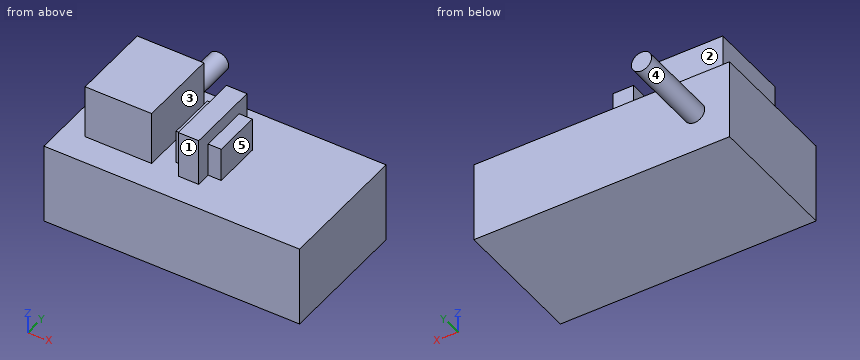
from build123d import *

# Parameters (mm, degrees)
F0_W     = 241.3
F0_H     = 76.2
F1_DEPTH = 127
F2_W     = 62.8207884729
F2_H     = 76.4612257481
F3_DEPTH = 50.8
F4_W     = 19.3203594536
F4_H     = 70.8669982851
F5_DEPTH = 44.45
F6_W     = 10.7880616561
F6_H     = 45.5669872463
F6_W_2   = 12.3340738937
F6_H_2   = 45.5182045698
F7_DEPTH = 31.75
F8_R     = 9.525
F9_DEPTH = 77.978


with BuildPart() as f1:
    # F0 (on Front) → F1 (new body)
    with BuildSketch(Plane.XZ):
        Rectangle(F0_W, F0_H)
    extrude(amount=-F1_DEPTH)

    # F2 (on face) → F3 (join)
    with BuildSketch(Plane.XY.offset(38.1)):
        with Locations((-68.2148206979, 66.0216137767)):
            Rectangle(F2_W, F2_H)
    extrude(amount=F3_DEPTH)

    # F4 (on face) → F5 (join)
    with BuildSketch(Plane.XY.offset(38.1)):
        with Locations((-0.7133577019, 61.1537639052)):
            Rectangle(F4_W, F4_H)
    extrude(amount=F5_DEPTH)

    # F6 (on face) → F7 (join)
    with BuildSketch(Plane.XY.offset(38.1)):
        with Locations((-15.7675682567, 62.2907597572)):
            Rectangle(F6_W, F6_H)
        with Locations((15.1138589717, 62.3151510954)):
            Rectangle(F6_W_2, F6_H_2)
    extrude(amount=F7_DEPTH)

    # F8 (on face) → F9 (join)
    with BuildSketch(Plane(origin=(0, 127, 0), x_dir=(-1, 0, 0), z_dir=(0, 1, 0))):
        with Locations((87.699372661, 0)):
            Circle(F8_R)
    extrude(amount=F9_DEPTH)


solid = f1.part
Work out the finished part from the listing and answer in its coordinate system (mm). Face numbers are marked on the shaded views. A direction names the side the tool comes from. Coordinates: 2 decimals unless noted, no trailing zeros. Write each loop counter-clockwise with the first axis right and the second up, starting at its lowest first coordinate (ties: lowest second). Pieces come first, ordered by that corner, then holes.
1. For the marked faces 1, 2, 3, 4 and 5, determine the directions among +Z, -Z, +X, -X, +Y, -Y from which every point of the face is accessible in a straight line to the end or side of a thin tool.
Results list:
face 1: +Z, +X, -X, -Y
face 2: +Z, +X, -X, +Y
face 3: +Z, +Y, -Y
face 4: +Y
face 5: +Z, +X, +Y, -Y
2. Consider line 1 along X through (y, z) = (66.5, 45.5); line 2 along X through (y, z) = (31.5, 81); line 3 along Y through (x, z) = (101, -9.5). Determine where each line is inside the solid, lowest interval first.
Results list:
line 1: x = -99.63 to -36.8, -21.16 to 21.28
line 2: x = -99.63 to -36.8, -10.37 to 8.95
line 3: y = 0 to 127
3. The part is cut by section C-C, the plane z = 0. Write down the section's boundary in (x, y).
Results list:
outline: (-120.65, 0) - (120.65, 0) - (120.65, 127) - (-78.17, 127) - (-78.17, 204.98) - (-97.22, 204.98) - (-97.22, 127) - (-120.65, 127) - close
4. The part is cut by section B-B, the plane x = -45. Write down the section's boundary in (y, z).
Results list:
outline: (0, -38.1) - (127, -38.1) - (127, 38.1) - (104.25, 38.1) - (104.25, 88.9) - (27.79, 88.9) - (27.79, 38.1) - (0, 38.1) - close
5. The part is cut by section A-A, the plane z = 56.5. Write down the section's boundary in (x, y).
Results list:
outline: (-99.63, 27.79) - (-36.8, 27.79) - (-36.8, 104.25) - (-99.63, 104.25) - close; (-21.16, 39.51) - (-10.37, 39.51) - (-10.37, 25.72) - (8.95, 25.72) - (8.95, 39.56) - (21.28, 39.56) - (21.28, 85.07) - (8.95, 85.07) - (8.95, 96.59) - (-10.37, 96.59) - (-10.37, 85.07) - (-21.16, 85.07) - close
6. Flat-ended cylindrical pins translate along their axes: pin 1 (15 mm diameter, centred on y = 48.5, z = 53.5, fed in from +X); pin 2 (15.5 mm diameter, centred on x = -2.5, y = 71, fed in from +Z); pin 3 (1 mm diameter, centred on x = 48, y = 61, fed in from +Z); pin 4 (6 mm diameter, centred on x = -20, z = 74, fed in from -Y). Find the tip coordinate at first contact, or state that the pin passes through.
Results list:
pin 1: stops at x = 21.28
pin 2: stops at z = 82.55
pin 3: stops at z = 38.1
pin 4: passes through
7. The part is cut by section D-D, the plane y = 48. Write down the section's boundary in (x, z), and give its area (3 significant figures).
Results list:
outline: (-120.65, -38.1) - (120.65, -38.1) - (120.65, 38.1) - (21.28, 38.1) - (21.28, 69.85) - (8.95, 69.85) - (8.95, 82.55) - (-10.37, 82.55) - (-10.37, 69.85) - (-21.16, 69.85) - (-21.16, 38.1) - (-36.8, 38.1) - (-36.8, 88.9) - (-99.63, 88.9) - (-99.63, 38.1) - (-120.65, 38.1) - close
area: 23,200 mm2
